from build123d import *

# Parameters (mm, degrees)
F0_R     = 3
F0_R_2   = 5.5
F1_DEPTH = 11
F2_R     = 3
F2_R_2   = 5.5
F3_DEPTH = 11
F4_R     = 3
F5_DEPTH = 12.5
F6_R     = 3
F7_DEPTH = 22.001


with BuildPart() as f1:
    # F0 (on Front) → F1 (new body, symmetric)
    with BuildSketch(Plane.XZ):
        Circle(F0_R)
        Circle(F0_R_2)
        Circle(F0_R, mode=Mode.SUBTRACT)
    extrude(amount=F1_DEPTH, both=True)

    # F2 (on Top) → F3 (join, symmetric)
    with BuildSketch(Plane.XY):
        with Locations((8, 0)):
            Circle(F2_R)
        with Locations((8, 0)):
            Circle(F2_R_2)
        with Locations((8, 0)):
            Circle(F2_R, mode=Mode.SUBTRACT)
    extrude(amount=F3_DEPTH, both=True)

    # F4 (on Front) → F5 (cut, symmetric)
    with BuildSketch(Plane.XZ):
        Circle(F4_R)
    extrude(amount=F5_DEPTH, both=True, mode=Mode.SUBTRACT)

    # F6 (on face) → F7 (cut, through all)
    with BuildSketch(Plane(origin=(0, 0, -11), x_dir=(1, 0, 0), z_dir=(0, 0, -1))):
        with Locations((8, 0)):
            Circle(F6_R)
    extrude(amount=-F7_DEPTH, mode=Mode.SUBTRACT)


solid = f1.part
Here's how the part is built. I have some questions about the finished solid (model axes, mm). A direction names the side the tool comes from. Give positions to 0.01 mm unless a question says otherwise; leave off trailing zeros. Write each loop counter-clockwise with the first axis right and the second up, starting at its lowest first coordinate (ties: lowest second). Pieces come first, ordered by that corner, then holes. Notation, with made-up numbers: (28.25, 11) -> (72.25, 11) arc R26 cw to (72.25, 43) -> close; hole circle Ø5 at (8.5, 64.25). An arc over 180 degrees is marked (long way). Use one line per item in the form item = value. Start each with the question number.
1. On a 3-axis mill with a long thin cutter (end or side, diameter ignored), from which of +Z, -Z, +X, -X, +Y, -Y can I reach the whole of each face in a straight line? I mean faces 1 (the face through (10.4, -2.4, -11)), 2 (the face through (-5.495, -0.154, 0.242)). Say none if no direction works.
2. Imagine slicing it at B-B on x = 0. List the corners of the cut face in (y, z) for me.
3. Will these pins go through, and if not, where does the flat tip stop? pin 1 Ø1 at (y, z) = (-1, 2) entering from +X; pin 2 Ø2 at (x, y) = (1, -3) entering from +Z; pin 3 Ø3 at (y, z) = (2.5, -8) entering from +X.
4. Thinking about a two-plate mould opening in X: for faces 3 (the face through (13.246, 1.652, 0.154)), 4 (the face through (2.4, 11, -2.4)), which applies, +X half, -X half, draft (parallel to the pull), parting line (faces both ways), or undercut?
5. Imagine slicing it at D-D on y = -4.5. List the corners of the cut face in (x, z) for me.
6. If I drill on L1, parallel to Z at x = 0, y = -6.5; L2, parallel to X at y = 0, z = -1, over which ranges is the centre line in solid material (lowest first)?
7. Imagine slicing it at A-A on y = 1. List the corners of the cut face in (x, z) for me, plus the area to 3 significant figures.
8. Imagine slicing it at C-C on z = 0. List the corners of the cut face in (x, y) for me.
Entries:
q1.face_1 = -Z, +X, -X, +Y, -Y
q1.face_2 = none
q2.outline = (-11, -5.5) -> (11, -5.5) -> (11, -3) -> (-11, -3) -> close; (-11, 3) -> (11, 3) -> (11, 5.5) -> (-11, 5.5) -> close
q3.pin_1 = 13.48
q3.pin_2 = 5.5
q3.pin_3 = 13.41
q4.face_3 = undercut
q4.face_4 = draft
q5.outline = (4.84, -11) -> (11.16, -11) -> (11.16, 11) -> (4.84, 11) -> (4.84, 2.62) arc R5.5 ccw (long way) to (4.84, -2.62) -> close; hole circle Ø6 at (0, 0)
q6.L1 = -5.5 to -3, 3 to 5.5
q6.L2 = -5.41 to -2.83, 2.83 to 5, 11 to 13.5
q7.outline = (2.59, -11) -> (5.17, -11) -> (5.17, 11) -> (2.59, 11) -> (2.59, 4.85) arc R5.5 ccw (long way) to (2.59, -4.85) -> close; (10.83, -11) -> (13.41, -11) -> (13.41, 11) -> (10.83, 11) -> close; hole circle Ø6 at (0, 0)
q7.area = 160 mm²
q8.outline = (-5.5, -11) -> (-3, -11) -> (-3, 11) -> (-5.5, 11) -> close; (3, -11) -> (5.5, -11) -> (5.5, -4.9) arc R5.5 ccw (long way) to (5.5, 4.9) -> (5.5, 11) -> (3, 11) -> close; hole circle Ø6 at (8, 0)
